Drawing for the job (mm, zero at the part's lowest x, y, z). Round coordinates to 2 decimals unless told otherwise and drop trailing zeros. Loops run counter-clockwise (first coordinate to the right, second up) from the corner with the lowest first, then second, coordinate; pieces in that order, holes last. Notation, with made-up numbers: (14.25, 85) -> (61.25, 85) arc R3 ccw to (61.25, 90) -> close; hole circle Ø9 at (85, 58.25). An arc over 180 degrees is marked (long way). Put each result on its own line as item: value. Start each with the question number.
Item 1: Cut at B-B, the plane x = 39. List the corners of the cut face in (y, z), plus the area to 3 significant figures.
Item 2: Drill centre lines: probe 1 along X at (y, z) = (112, 1); probe 2 along Y at (x, z) = (16.5, 2); probe 3 along X at (y, z) = (95, 4.6). Where is each one in solid material? Low to high. Write a range as [from, to].
Item 3: Cut at A-A, the plane z = 1.25. List the corners of the cut face in (x, y), plus the area to 3 significant figures.
Item 4: Cut at C-C, the plane y = 37. List the corners of the cut face in (x, z), plus the area to 3 significant figures.
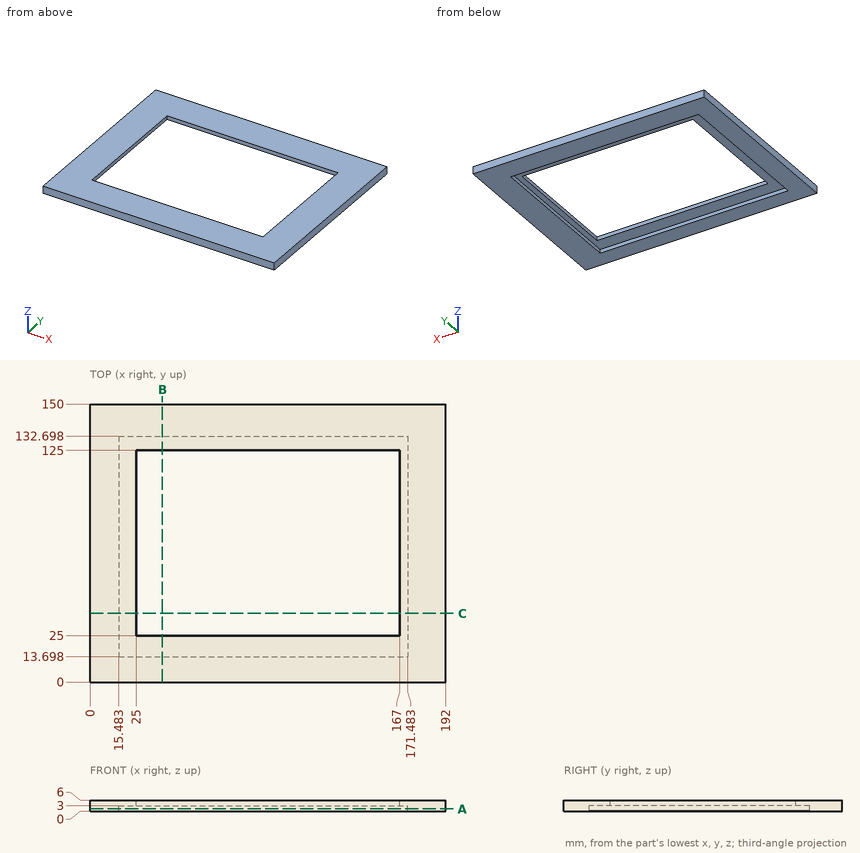
Reply:
1. outline: (0, 0) -> (13.7, 0) -> (13.7, 3) -> (25, 3) -> (25, 6) -> (0, 6) -> close; (125, 3) -> (132.7, 3) -> (132.7, 0) -> (150, 0) -> (150, 6) -> (125, 6) -> close
1. area: 243 mm^2
2. probe 1: x = [0, 15.48], [171.48, 192]
2. probe 2: y = [0, 13.7], [132.7, 150]
2. probe 3: x = [0, 25], [167, 192]
3. outline: (0, 0) -> (192, 0) -> (192, 150) -> (0, 150) -> close; hole (15.48, 13.7) -> (171.48, 13.7) -> (171.48, 132.7) -> (15.48, 132.7) -> close
3. area: 10,200 mm^2
4. outline: (0, 0) -> (15.48, 0) -> (15.48, 3) -> (25, 3) -> (25, 6) -> (0, 6) -> close; (167, 3) -> (171.48, 3) -> (171.48, 0) -> (192, 0) -> (192, 6) -> (167, 6) -> close
4. area: 258 mm^2
